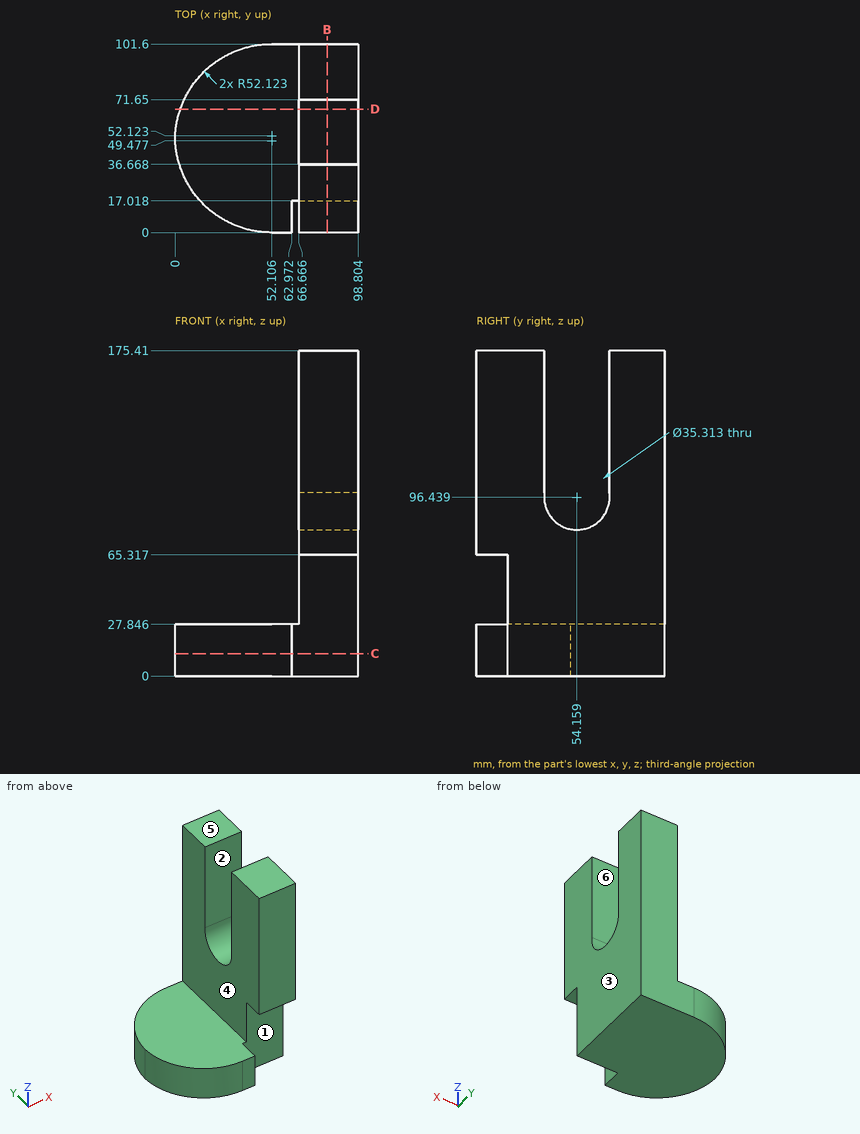
Input: dimensioned drawing with shaded views. Units: mm. Origin: part minimum x, y, z. A direction names the side the tool comes from. Coordinates: 2 decimals unless noted, no trailing zeros. Write each loop counter-clockwise with the first axis right and the second up, starting at its lowest first coordinate (ties: lowest second). Pieces come first, ordered by that corner, then holes. Notation, with made-up numbers: M 53,-34.75 L 67,-34.75 A30 cw 67,-8.75 Z; hole C 83,71 d4. An arc over 180 degrees is marked long. Answer as CSV lines item,"result". Start each with the question number.
Q1. Cut plane B-B on x = 82. Return the cut outline in (y, z), then the cut area to 3 significant figures.
Q2. Line query: line 1 (Y direction, x = 88.5, z = 119.5); line 2 (X direction, y = 75.5, z = 104) (1 decimal); line 3 (Y direction, x = 92.5, z = 36). Output: solid intervals per line, ascending. Write a range as from..to.
Q3. Reachability of the marked faces 4, 5 and 6 from +Z, -Z, +X, -X, +Y, -Y: full face, straight path, thin tool, end or side. Return the list, or none.
Q4. Pin query (flat end, axial travel): P1, Ø10, axis at x = 64, z = 82, coming from the -Y side; P2, Ø5, axis at y = 5, z = 10, coming from the +X side; P3, Ø20, axis at x = 38, y = 62.5, coming from the +Z side; P4, Ø10, axis at y = 22, z = 117.5, coming from the -X side. Return the tip coordinate at first contact, or that it passes through.
Q5. Cut plane D-D on y = 66.5. Return the cut outline in (x, z) (1 decimal).
Q6. Cut plane C-C on z = 12. Return the cut outline in (x, y) (1 decimal), then the cut area to 3 significant figures.
Q7. Mould query, pull axis Y, two halves, no side actions, for the marked faces 1, 2 and 3. Classes: released by +Y, released by -Y, zero draft, split by the parting line, or undercut.
Findings below:
1,outline,"M 0,65.32 L 17.02,65.32 L 17.02,0 L 101.6,0 L 101.6,175.41 L 71.65,175.41 L 71.65,98.85 A17.66 cw long 36.67,98.85 L 36.67,175.41 L 0,175.41 Z"
1,area,"13,500 mm2"
2,line 1,"y = 0..36.67, 71.65..101.6"
2,line 2,"x = 66.7..98.8"
2,line 3,"y = 17.02..101.6"
3,face 4,"+Z, -X, +Y, -Y"
3,face 5,"+Z, +X, -X, +Y, -Y"
3,face 6,"+Z, +X, -X"
4,P1,"stops at y = 0"
4,P2,"stops at x = 62.97"
4,P3,"stops at z = 27.85"
4,P4,"stops at x = 66.67"
5,outline,"M 2.8,0 L 98.8,0 L 98.8,83.8 L 66.7,83.8 L 66.7,27.8 L 2.8,27.8 Z"
6,outline,"M 0,50.8 A52.1 ccw 52.1,0 L 63,0 L 63,17 L 98.8,17 L 98.8,101.6 L 52.1,101.6 A52.1 ccw Z"
6,area,"8,260 mm2"
7,face 1,"released by -Y"
7,face 2,"undercut"
7,face 3,"zero draft"
